Part model, mm, in its own coordinate system. A direction names the side the tool comes from. Round coordinates to 2 decimals unless told otherwise and drop trailing zeros. Order: outer loops, then holes, each group sorted by start corner. A loop starts at its lowest first (then second) coordinate and runs counter-clockwise, first axis right, second up. Notation, with made-up numbers: (57, 25) - (89, 25) arc R17 cw to (89, 42) - close; hole circle Ø7 at (-3.75, 39.5). An arc over 180 degrees is marked (long way). Answer as a JSON object with one key per item and string values.
```python
from build123d import *

# Parameters (mm, degrees)
F0_W     = 285
F0_H     = 80
F1_DEPTH = 180
F2_W     = 265
F2_H     = 160
F3_DEPTH = 70
F5_DEPTH = 285.001
F7_DEPTH = 70
F8_SIZE2 = 50
F8_SIZE  = 50


with BuildPart() as f1:
    # F0 (on Front) → F1 (new body)
    with BuildSketch(Plane.XZ):
        with Locations((142.5, 40)):
            Rectangle(F0_W, F0_H)
    extrude(amount=-F1_DEPTH)

    # F2 (on face) → F3 (cut)
    with BuildSketch(Plane.XY.offset(80)):
        with Locations((142.5, 90)):
            Rectangle(F2_W, F2_H)
    extrude(amount=-F3_DEPTH, mode=Mode.SUBTRACT)

    # F4 (on face) → F5 (cut, through all)
    with BuildSketch(Plane.YZ.offset(285)):
        with BuildLine():
            Line((115, 66), (65, 66))
            ThreePointArc((65, 66), (54, 55), (65, 44))
            Line((65, 44), (115, 44))
            ThreePointArc((115, 44), (126, 55), (115, 66))
        make_face()
    extrude(amount=-F5_DEPTH, mode=Mode.SUBTRACT)

    # F6 (on face) → F7 (join)
    with BuildSketch(Plane.XY.offset(80)):
        Polygon((100, 170), (90, 170), (90, 95), (11, 95), (11, 85), (90, 85), (90, 10), (100, 10), (100, 85), (185, 85), (185, 10), (195, 10), (195, 85), (274, 85), (274, 95), (195, 95), (195, 170), (185, 170), (185, 95), (100, 95), align=None)
    extrude(amount=-F7_DEPTH)

    # F8
    f8_edges = [f1.edges().sort_by_distance(p)[0] for p in [
        (11, 90, 80),
        (274, 90, 80),
    ]]
    chamfer(f8_edges, length=F8_SIZE, length2=F8_SIZE2)


solid = f1.part
```
Item 1: Cut at C-C (y = 51). Write the cut outline in (x, z), plus the area to 3 significant figures.
Taken from the geometry:
{"outline": "(0, 0) - (285, 0) - (285, 80) - (275, 80) - (275, 10) - (195, 10) - (195, 80) - (185, 80) - (185, 10) - (100, 10) - (100, 80) - (90, 80) - (90, 10) - (10, 10) - (10, 80) - (0, 80) - close", "area": "5,650 mm2"}
Item 2: Two-plate mould, pull along X, no slides. Class faces 4 (the cylindrical face through (5, 54, 55)), 5 (the flat face through (249, 90, 55)): pulls with the +X half, pulls with the -X half, needs draft (parallel to the pull), parting line crosses it, or undercut.
Taken from the geometry:
{"face 4": "needs draft", "face 5": "undercut"}
Item 3: Tool access for faces 1 (the flat face through (280, 90, 66)), 2 (the flat face through (5, 90, 44)), 3 (the flat face through (185, 133, 45)): list every direction of +Z, -Z, +X, -X, +Y, -Y with a clear straight run to the whole face (end or side of a thin tool).
Taken from the geometry:
{"face 1": "+X", "face 2": "-X", "face 3": "+Z"}
Item 4: Cut at D-D (z = 55). State how many separate pieces and enclosed holes the cut face has, plus the area to 3 significant figures.
Taken from the geometry:
{"separate pieces": "1", "enclosed holes": "2", "area": "12,600 mm2"}
Item 5: Cut at B-B (x = 230.5). Write the cut outline in (y, z).
Taken from the geometry:
{"outline": "(0, 0) - (180, 0) - (180, 80) - (170, 80) - (170, 10) - (95, 10) - (95, 73.5) - (85, 73.5) - (85, 10) - (10, 10) - (10, 80) - (0, 80) - close"}
Item 6: Cut at A-A (z = 17). Write the cut outline in (x, y).
Taken from the geometry:
{"outline": "(0, 0) - (285, 0) - (285, 180) - (0, 180) - close; hole (10, 10) - (90, 10) - (90, 85) - (11, 85) - (11, 95) - (90, 95) - (90, 170) - (10, 170) - close; hole (100, 10) - (185, 10) - (185, 85) - (100, 85) - close; hole (100, 95) - (185, 95) - (185, 170) - (100, 170) - close; hole (195, 10) - (275, 10) - (275, 170) - (195, 170) - (195, 95) - (274, 95) - (274, 85) - (195, 85) - close"}
Item 7: Drop a flat-ended pin along its axis: P1, Ø2, axis at x = 179.5, y = 101.5, coming from the +Z side. Give the stop position or say it passes through.
Taken from the geometry:
{"P1": "z = 10"}
Item 8: Probe L1, parallel to Y at x = 181, z = 27; L2, parallel to X at y = 82, z = 40.5; L3, parallel to X at y = 76, z = 64. List the from-to ranges inside material, lowest first. Write a range as from..to.
Taken from the geometry:
{"L1": "0..10, 85..95, 170..180", "L2": "0..10, 90..100, 185..195, 275..285", "L3": "90..100, 185..195"}
